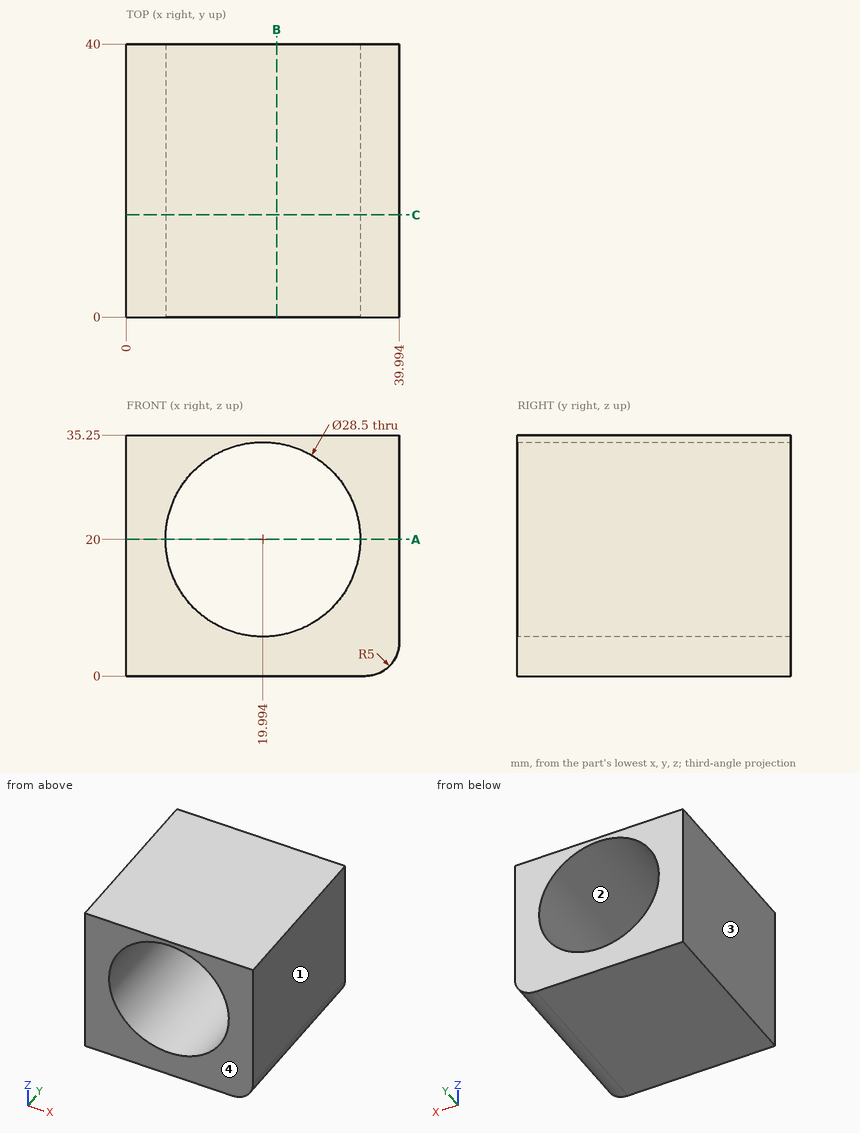
Could you check a few things on this drawing? It's one solid part, dimensions in mm from its lowest x, y, z. Round coordinates to 2 decimals unless told otherwise and drop trailing zeros. Write each loop counter-clockwise with the first axis right and the second up, starting at its lowest first coordinate (ties: lowest second). Pieces come first, ordered by that corner, then holes. Notation, with made-up numbers: (55.5, -31.75) -> (80.5, -31.75) arc R13 ccw to (80.5, -23.75) -> close; hole circle Ø8 at (33, 17). An arc over 180 degrees is marked (long way). Use a Markdown table: item, result.
1. We'd pull the mould along X, two halves only. Please class the marked faces 1, 2, 3 and 4: +X half, -X half, draft (parallel to the pull), parting line (faces both ways), or undercut.
Answer key:
| item | result |
|---|---|
| face 1 | +X half |
| face 2 | undercut |
| face 3 | -X half |
| face 4 | draft |
2. If we section it at A-A (z = 20): List the corners of the cut face in (x, y) for me.
Answer key:
| item | result |
|---|---|
| outline | (0, 0) -> (5.74, 0) -> (5.74, 40) -> (0, 40) -> close; (34.24, 0) -> (39.99, 0) -> (39.99, 40) -> (34.24, 40) -> close |
3. If we section it at B-B (x = 22): List the corners of the cut face in (y, z) for me, then the cut area to 3 significant figures.
Answer key:
| item | result |
|---|---|
| outline | (0, 0) -> (40, 0) -> (40, 5.89) -> (0, 5.89) -> close; (0, 34.11) -> (40, 34.11) -> (40, 35.25) -> (0, 35.25) -> close |
| area | 281 mm^2 |
4. Please list where these lines run through material, in increasing order: probe 1 along X at (y, z) = (14.5, 20); probe 2 along Z at (x, y) = (25.5, 24.5); probe 3 along Z at (x, y) = (23, 21.5).
Answer key:
| item | result |
|---|---|
| probe 1 | x = 0 to 5.74, 34.24 to 39.99 |
| probe 2 | z = 0 to 6.86, 33.14 to 35.25 |
| probe 3 | z = 0 to 6.07, 33.93 to 35.25 |
5. If we section it at C-C (y = 15): List the corners of the cut face in (x, z) for me.
Answer key:
| item | result |
|---|---|
| outline | (0, 0) -> (34.99, 0) arc R5 ccw to (39.99, 5) -> (39.99, 35.25) -> (0, 35.25) -> close; hole circle Ø28.5 at (19.99, 20) |
